```python
from build123d import *

# Parameters (mm, degrees)
F1_DEPTH = 38.1
F2_R     = 6.35
F3_R     = 6.35
F5_D     = 5.1054
F6_R     = 3.175
F7_R     = 3.175


with BuildPart() as f1:
    # F0 (on Front) → F1 (new body, symmetric)
    with BuildSketch(Plane.XZ):
        Polygon((-27.8152357787, 1.5875), (-27.8152357787, -1.5875), (27.8152357787, -1.5875), (27.8152357787, 1.5875), (27.8152357787, 62.5623540473), (73.2854913984, 62.5623540473), (73.2899605753, 65.7373509019), (27.8197049557, 65.7373509019), (24.6402357787, 65.7373509019), (24.6402357787, 62.5623540473), (24.6402357787, 9.6064366907), (24.6402357787, 1.5875), align=None)
    extrude(amount=F1_DEPTH, both=True)

    # F2
    f2_edges = [f1.edges().sort_by_distance(p)[0] for p in [
        (-27.815236, -38.1, 0),
    ]]
    fillet(f2_edges, radius=F2_R)

    # F3
    f3_edges = [f1.edges().sort_by_distance(p)[0] for p in [
        (73.287726, 38.1, 64.149852),
        (73.287726, -38.1, 64.149852),
        (-27.815236, 38.1, 0),
    ]]
    fillet(f3_edges, radius=F3_R)

    # F5 (through all)
    with Locations(Plane.XY.offset(1.5875)):
        with Locations((-8.7652357787, 19.05), (-8.7652357787, -19.05)):
            Hole(F5_D / 2)

    # F6
    f6_edges = [f1.edges().sort_by_distance(p)[0] for p in [
        (24.640236, 0, 65.737351),
        (27.815236, 0, -1.5875),
    ]]
    fillet(f6_edges, radius=F6_R)

    # F7
    f7_edges = [f1.edges().sort_by_distance(p)[0] for p in [
        (27.815236, 0, 62.562354),
        (24.640236, 0, 1.5875),
    ]]
    fillet(f7_edges, radius=F7_R)


solid = f1.part
```
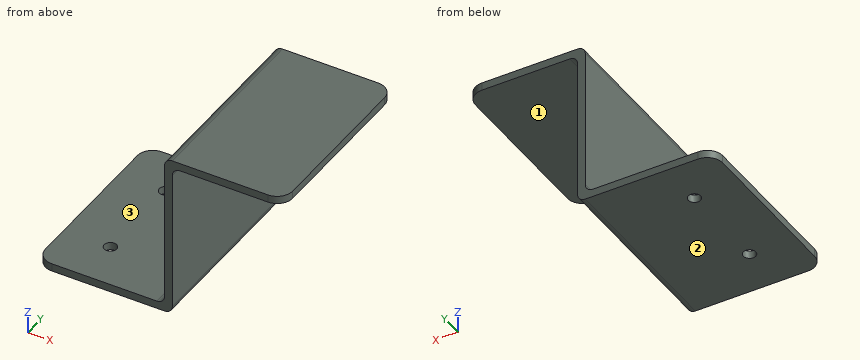
The listing builds one solid part. Answer for the finished solid, in the listing's coordinates (mm). Face numbers are marked on the shaded views. A direction names the side the tool comes from. Round coordinates to 2 decimals unless told otherwise and drop trailing zeros. Loops run counter-clockwise (first coordinate to the right, second up) from the corner with the lowest first, then second, coordinate; pieces in that order, holes last.
Q1. Given pin 1 Ø10 at (y, z) = (-11.5, 15.5) entering from -X; pin 2 Ø15 at (x, y) = (-8, -7) entering from +Z, each flat-ended and moving along its own axis, determine where each tip first touches the part or whether it passes through.
Q2. Which of the six approach directions +Z, -Z, +X, -X, +Y, -Y give full straight-line access (tool end or side, diameter ignored) to the marked faces 1, 2 and 3?
Q3. Find the intervals of material crossed by line 1 (Z direction, x = 1.5, y = 14.5); line 2 (X direction, y = 16, z = 48); line 3 (X direction, y = 19, z = 0), in increasing order.
Q4. Section D-D, the plane z = 27 is taken. Determine the outline of the cut face in (x, y), then the cut area to 3 significant figures.
Q5. Section B-B, the plane x = -7.5 is taken. Determine the outline of the cut face in (y, z), then the cut area to 3 significant figures.
Completed:
1. pin 1: stops at x = 24.64
1. pin 2: stops at z = 1.59
2. face 1: -Z, +X, +Y, -Y
2. face 2: -Z, +X, -X, +Y, -Y
2. face 3: +Z, -X, +Y, -Y
3. line 1: z = -1.59 to 1.59
3. line 2: x = 24.64 to 27.82
3. line 3: x = -27.82 to -11.32, -6.21 to 27.39
4. outline: (24.64, -38.1) - (27.82, -38.1) - (27.82, 38.1) - (24.64, 38.1) - close
4. area: 242 mm2
5. outline: (-38.1, -1.59) - (-21.27, -1.59) - (-21.27, 1.59) - (-38.1, 1.59) - close; (-16.83, -1.59) - (16.83, -1.59) - (16.83, 1.59) - (-16.83, 1.59) - close; (21.27, -1.59) - (38.1, -1.59) - (38.1, 1.59) - (21.27, 1.59) - close
5. area: 214 mm2
